Input: dimensioned drawing with shaded views. Units: mm. Origin: part minimum x, y, z. A direction names the side the tool comes from. Round coordinates to 2 decimals unless told otherwise and drop trailing zeros. Write each loop counter-clockwise with the first axis right and the second up, starting at its lowest first coordinate (ties: lowest second). Pieces come first, ordered by that corner, then holes. Notation, with made-up numbers: (62, -39) - (79, -39) arc R6 ccw to (79, -34) - close; hole circle Ø8 at (38.5, -21.5). An arc over 180 degrees is marked (long way). Write item = value, one per line. Start each with the question number.
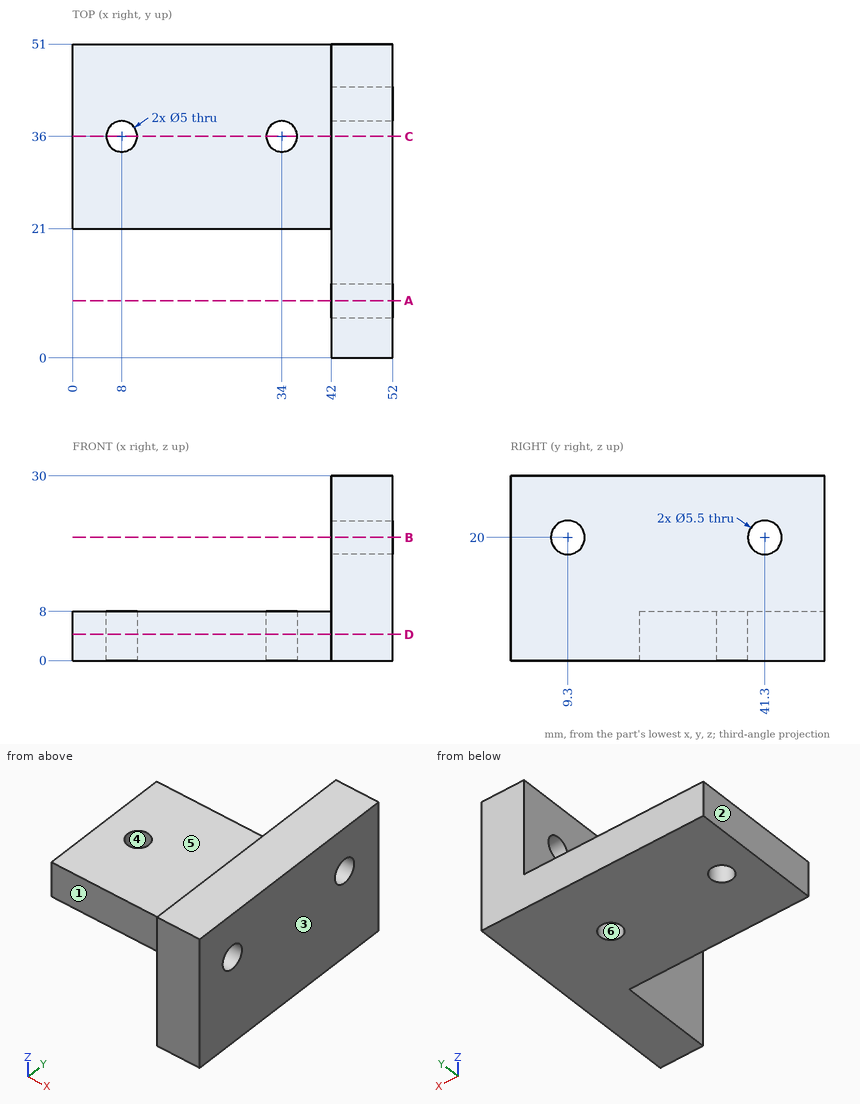
(1) Pull-direction query (X, two-part tool) for the marked faces 3, 4, 5 and 6; classes: +X half, -X half, draft (parallel to the pull), parting line (faces both ways), or undercut.
(2) Contact query for flat-ended pins moving along their axis: P1, Ø8, axis at x = 6, y = 20.5, coming from the +Z side; P2, Ø6, axis at x = 32, z = 6, coming from the -Y side. Output: stop coordinate, or through.
(3) Section C-C (y = 36). Return the cut outline in (x, z), plus the area to 3 significant figures.
(4) Section D-D (z = 4.25). Return the cut outline in (x, y).
(5) Reachability of the marked faces 1 and 2 from +Z, -Z, +X, -X, +Y, -Y: full face, straight path, thin tool, end or side. Return the list, or none.
(6) Ray query, L1, parallel to Y at x = 48.75, z = 20; L2, parallel to X at y = 35.5, z = 2.25; L3, parallel to Y at x = 34, z = 4.5. Return the intervals inside material, ascending. Write a range as from..to.
(7) Section A-A (y = 9.3). Return the cut outline in (x, z).
(8) Section B-B (z = 20). Return the cut outline in (x, y).
Solution:
q1.face_3 = +X half
q1.face_4 = undercut
q1.face_5 = draft
q1.face_6 = undercut
q2.P1 = 8
q2.P2 = 21
q3.outline = (0, 0) - (5.5, 0) - (5.5, 8) - (0, 8) - close; (10.5, 0) - (31.5, 0) - (31.5, 8) - (10.5, 8) - close; (36.5, 0) - (52, 0) - (52, 30) - (42, 30) - (42, 8) - (36.5, 8) - close
q3.area = 556 mm^2
q4.outline = (0, 21) - (42, 21) - (42, 0) - (52, 0) - (52, 51) - (0, 51) - close; hole circle Ø5 at (8, 36); hole circle Ø5 at (34, 36)
q5.face_1 = +Z, -Z, -X, -Y
q5.face_2 = +Z, -Z, -X, +Y, -Y
q6.L1 = 0..6.55, 12.05..38.55, 44.05..51
q6.L2 = 0..5.55, 10.45..31.55, 36.45..52
q6.L3 = 21..33.5, 38.5..51
q7.outline = (42, 0) - (52, 0) - (52, 17.25) - (42, 17.25) - close; (42, 22.75) - (52, 22.75) - (52, 30) - (42, 30) - close
q8.outline = (42, 0) - (52, 0) - (52, 6.55) - (42, 6.55) - close; (42, 12.05) - (52, 12.05) - (52, 38.55) - (42, 38.55) - close; (42, 44.05) - (52, 44.05) - (52, 51) - (42, 51) - close
